from build123d import *

# Parameters (mm, degrees)
SKETCH1_R           = 1.5
BOSS_EXTRUDE1_DEPTH = 15
BOSS_EXTRUDE2_DEPTH = 85
SKETCH3_R           = 11
BOSS_EXTRUDE3_DEPTH = 2
SKETCH4_R           = 2.5
BOSS_EXTRUDE4_DEPTH = 22
CUT_EXTRUDE1_DEPTH  = 15
SKETCH6_W           = 42.3
SKETCH6_H           = 75
BOSS_EXTRUDE5_DEPTH = 30
SKETCH7_W           = 42.3
SKETCH7_H           = 32.7
BOSS_EXTRUDE6_DEPTH = 30
FILLET1_R           = 5


with BuildPart() as part:
    # Sketch1 → Boss-Extrude1 (new body)
    with BuildSketch(Plane(origin=(0, 0, 0), x_dir=(1, 0, 0), z_dir=(0, 1, 0))):
        Polygon((5.65, 0), (36.65, 0), (42.3, 5.65), (42.3, 36.65), (36.65, 42.3), (5.65, 42.3), (0, 36.65), (0, 5.65), align=None)
        with Locations((5.65, 5.65)):
            Circle(SKETCH1_R, mode=Mode.SUBTRACT)
        with Locations((36.65, 5.65)):
            Circle(SKETCH1_R, mode=Mode.SUBTRACT)
        with Locations((36.65, 36.65)):
            Circle(SKETCH1_R, mode=Mode.SUBTRACT)
        with Locations((5.65, 36.65)):
            Circle(SKETCH1_R, mode=Mode.SUBTRACT)
    extrude(amount=BOSS_EXTRUDE1_DEPTH)

    # Sketch2 → Boss-Extrude2 (add)
    with BuildSketch(Plane.XZ):
        Polygon((5.65, 0), (0, -5.65), (0, -36.65), (5.65, -42.3), (36.65, -42.3), (42.3, -36.65), (42.3, -5.65), (36.65, 0), align=None)
    extrude(amount=BOSS_EXTRUDE2_DEPTH)

    # Sketch3 → Boss-Extrude3 (add)
    with BuildSketch(Plane(origin=(0, 15, 0), x_dir=(1, 0, 0), z_dir=(0, 1, 0))):
        with Locations((21.15, 21.15)):
            Circle(SKETCH3_R)
    extrude(amount=BOSS_EXTRUDE3_DEPTH)

    # Sketch4 → Boss-Extrude4 (add)
    with BuildSketch(Plane(origin=(0, 17, 0), x_dir=(1, 0, 0), z_dir=(0, 1, 0))):
        with Locations((21.15, 21.15)):
            Circle(SKETCH4_R)
    extrude(amount=BOSS_EXTRUDE4_DEPTH)

    # Sketch5 → Cut-Extrude1 (cut)
    with BuildSketch(Plane(origin=(0, 39, 0), x_dir=(1, 0, 0), z_dir=(0, 1, 0))):
        with BuildLine():
            Line((19.65, 23.15), (22.65, 23.15))
            ThreePointArc((22.65, 23.15), (21.15, 23.65), (19.65, 23.15))
        make_face()
    extrude(amount=-CUT_EXTRUDE1_DEPTH, mode=Mode.SUBTRACT)

    # Sketch6 → Boss-Extrude5 (add)
    with BuildSketch(Plane.XZ.offset(85)):
        with Locations((21.15, -4.8)):
            Rectangle(SKETCH6_W, SKETCH6_H)
    extrude(amount=BOSS_EXTRUDE5_DEPTH)

    # Sketch7 → Boss-Extrude6 (add)
    with BuildSketch(Plane(origin=(0, -85, 0), x_dir=(1, 0, 0), z_dir=(0, 1, 0))):
        with Locations((21.15, -16.35)):
            Rectangle(SKETCH7_W, SKETCH7_H)
    extrude(amount=BOSS_EXTRUDE6_DEPTH)

    # Fillet1
    fillet1_edges = [part.edges().sort_by_distance(p)[0] for p in [
        (21.15, -55, 32.7),
        (42.3, -85, 32.7),
        (0, -85, 32.7),
        (42.3, -115, -4.8),
        (21.15, -115, 32.7),
        (0, -115, -4.8),
    ]]
    fillet(fillet1_edges, radius=FILLET1_R)


solid = part.part
Source: CAD feature listing. Evaluate the final solid. Frame: model axes, mm. A direction names the side the tool comes from. Give positions to 0.01 mm unless a question says otherwise; leave off trailing zeros. Write each loop counter-clockwise with the first axis right and the second up, starting at its lowest first coordinate (ties: lowest second). Pieces come first, ordered by that corner, then holes. Notation, with made-up numbers: (66, -19) -> (103, -19) arc R34 cw to (103, 13) -> close; hole circle Ø3 at (2.25, -38). An arc over 180 degrees is marked (long way). Return JSON: item names as keys, results as strings. Group by question number.
1. Section A-A, the plane y = 8.5. Output: boundary loops of the cut face in (x, z).
2. Mould query, pull axis Z, two halves, no side actions, for faces 6 (the face through (21, -49, -42.3)), 7 (the face through (2, -85, -2)), 8 (the face through (0, -62, -7)). Classes: +Z half, -Z half, draft (parallel to the pull), parting line (faces both ways), or undercut.
3. Section B-B, the plane y = -30. Output: boundary loops of the cut face in (x, z).
4. Access query for faces 1 (the face through (39.44, -34.3, -39.51)), 2 (the face through (2, -85, -41)), 3 (the face through (21, 32, -23.15)), 4 (the face through (37, 0, -6)), 5 (the face through (21, -20, 0)). Directions: +Z, -Z, +X, -X, +Y, -Y. A direction counts if a zero-diameter tool reaches every point of the face in a straight line with its end or side. Return the directions, or none.
5. Material intervals for line 1 (Z direction, x = 5.65, y = 4.5); line 2 (X direction, y = 7, z = -5.65); line 3 (X direction, y = 7, z = -5), sorted ascending. Write a range as from..to.
6. Pin query (flat end, axial travel): pin 1 Ø10 at (y, z) = (-56.5, -10) entering from -X; pin 2 Ø4 at (x, z) = (36.65, -5.65) entering from +Y; pin 3 Ø3 at (x, z) = (12.5, -21) entering from +Y; pin 4 Ø1.5 at (x, z) = (29.5, 20) entering from +Y. Return the tip coordinate at first contact, or that it passes through.
7. Section C-C, the plane z = -21.15. Output: boundary loops of the cut face in (x, y).
8. Section D-D, the plane x = 16. Output: boundary loops of the cut face in (y, z).
Determined:
{
 "1": {"outline": "(0, -36.65) -> (5.65, -42.3) -> (36.65, -42.3) -> (42.3, -36.65) -> (42.3, -5.65) -> (36.65, 0) -> (5.65, 0) -> (0, -5.65) -> close; hole circle Ø3 at (5.65, -36.65); hole circle Ø3 at (5.65, -5.65); hole circle Ø3 at (36.65, -36.65); hole circle Ø3 at (36.65, -5.65)"},
 "2": {"face 6": "-Z half", "face 7": "undercut", "face 8": "draft"},
 "3": {"outline": "(0, -36.65) -> (5.65, -42.3) -> (36.65, -42.3) -> (42.3, -36.65) -> (42.3, -5.65) -> (36.65, 0) -> (5.65, 0) -> (0, -5.65) -> close"},
 "4": {"face 1": "-Z, +X, +Y", "face 2": "-Z, -X, +Y", "face 3": "-Z, +X, -X, +Y", "face 4": "+Y", "face 5": "+Z, +X, -X, +Y"},
 "5": {"line 1": "z = -42.3..-38.15, -35.15..-7.15, -4.15..0", "line 2": "x = 0..4.15, 7.15..35.15, 38.15..42.3", "line 3": "x = 0.65..4.3, 7..35.3, 38..41.65"},
 "6": {"pin 1": "stops at x = 0", "pin 2": "stops at y = 15", "pin 3": "stops at y = 17", "pin 4": "stops at y = -55"},
 "7": {"outline": "(0, -110) arc R5 ccw to (5, -115) -> (37.3, -115) arc R5 ccw to (42.3, -110) -> (42.3, 15) -> (32.15, 15) -> (32.15, 17) -> (23.65, 17) -> (23.65, 39) -> (18.65, 39) -> (18.65, 17) -> (10.15, 17) -> (10.15, 15) -> (0, 15) -> close"},
 "8": {"outline": "(-115, -42.3) -> (15, -42.3) -> (15, -30.87) -> (17, -30.87) -> (17, -11.43) -> (15, -11.43) -> (15, 0) -> (-55, 0) -> (-55, 27.7) arc R5 ccw to (-60, 32.7) -> (-110, 32.7) arc R5 ccw to (-115, 27.7) -> close"}
}
